Read the model definition and answer for the solid it produces. Units are mm, in the model's axes. A direction names the side the tool comes from. Coordinates: 2 decimals unless noted, no trailing zeros. Use a Markdown table: item, result.
from build123d import *

# Parameters (mm, degrees)
BOSS_EXTRUDE1_DEPTH = 11.1125
SKETCH2_R           = 12
CUT_EXTRUDE1_DEPTH  = 6
SKETCH3_R           = 10
CUT_EXTRUDE2_DEPTH  = 136.768702671
SKETCH4_R           = 3.2639
CUT_EXTRUDE3_DEPTH  = 137.09051503
SKETCH5_R           = 9.525
CUT_EXTRUDE4_DEPTH  = 4.7625
SKETCH6_R           = 2.778125
CUT_EXTRUDE5_DEPTH  = 38.1


with BuildPart() as part:
    # Sketch1 → Boss-Extrude1 (new body)
    with BuildSketch(Plane(origin=(-18.0375, 0, 0), x_dir=(0, 0, -1), z_dir=(1, 0, 0))):
        Polygon((-47.625, -127), (-47.625, 19.726920908), (-19.726920908, 47.625), (19.726920908, 47.625), (47.625, 19.726920908), (47.625, -127), align=None)
    extrude(amount=-BOSS_EXTRUDE1_DEPTH)

    # Sketch2 → Cut-Extrude1 (cut)
    with BuildSketch(Plane(origin=(-18.0375, 0, 0), x_dir=(0, 0, -1), z_dir=(1, 0, 0))):
        with Locations(Location((0, 0, 0), (0, 0, 90))):
            Circle(SKETCH2_R)
    extrude(amount=-CUT_EXTRUDE1_DEPTH, mode=Mode.SUBTRACT)

    # Sketch3 → Cut-Extrude2 (cut, through all)
    with BuildSketch(Plane(origin=(-24.0375, 0, 0), x_dir=(0, 0, -1), z_dir=(1, 0, 0))):
        with Locations(Location((0, 0, 0), (0, 0, 90))):
            Circle(SKETCH3_R)
    extrude(amount=-CUT_EXTRUDE2_DEPTH, mode=Mode.SUBTRACT)

    # Sketch4 → Cut-Extrude3 (cut, through all)
    with BuildSketch(Plane.ZY.offset(29.15)):
        with Locations((0, -31.75)):
            Circle(SKETCH4_R)
        with Locations((31.75, 0)):
            Circle(SKETCH4_R)
        with Locations((-31.75, 0)):
            Circle(SKETCH4_R)
        with Locations((0, 31.75)):
            Circle(SKETCH4_R)
    extrude(amount=-CUT_EXTRUDE3_DEPTH, mode=Mode.SUBTRACT)

    # Sketch5 → Cut-Extrude4 (cut)
    with BuildSketch(Plane(origin=(-18.0375, 0, 0), x_dir=(0, 0, -1), z_dir=(1, 0, 0))):
        with Locations(Location((-31.75, 0, 0), (0, 0, 90))):
            Circle(SKETCH5_R)
        with Locations(Location((0, 31.75, 0), (0, 0, 90))):
            Circle(SKETCH5_R)
        with Locations(Location((31.75, 0, 0), (0, 0, 90))):
            Circle(SKETCH5_R)
        with Locations(Location((0, -31.75, 0), (0, 0, 90))):
            Circle(SKETCH5_R)
    extrude(amount=-CUT_EXTRUDE4_DEPTH, mode=Mode.SUBTRACT)

    # Sketch6 → Cut-Extrude5 (cut)
    with BuildSketch(Plane.XZ.offset(127)):
        with Locations((-23.59375, 0)):
            Circle(SKETCH6_R)
        with Locations((-23.59375, 38.1)):
            Circle(SKETCH6_R)
        with Locations((-23.59375, -38.1)):
            Circle(SKETCH6_R)
    extrude(amount=-CUT_EXTRUDE5_DEPTH, mode=Mode.SUBTRACT)


solid = part.part
(1) Straight lines are drawn through the part: L1, parallel to Z at x = -21.4, y = 0 (3 decimals); L2, parallel to Z at x = -23, y = 0.5 (3 decimals); L3, parallel to X at y = 28, z = 6. For each, find the intervals that lie inside material, in ascending order.
Report:
| item | result |
|---|---|
| L1 | z = -47.625 to -41.275, -22.225 to -12, 12 to 22.225, 41.275 to 47.625 |
| L2 | z = -47.625 to -34.975, -28.525 to -11.99, 11.99 to 28.525, 34.975 to 47.625 |
| L3 | x = -29.15 to -22.8 |
(2) A cutting plane is placed at A-A, the plane z = 0. Count the separate pieces of the cut face and the enclosed holes in it, and give its area (3 significant figures).
Report:
| item | result |
|---|---|
| separate pieces | 4 |
| enclosed holes | 0 |
| area | 1,220 mm² |
(3) Each of these flat-tipped pins is pushed along its axis until it touches: P1, Ø22, axis at y = 0, z = -31.75, coming from the -X side; P2, Ø3.5, axis at x = -23.59, z = 38.1, coming from the +Y side; P3, Ø5.5, axis at y = 4, z = 34, coming from the +X side; P4, Ø6, axis at x = -20, z = -33, coming from the +Y side. Where does it stop, or does it pass through?
Report:
| item | result |
|---|---|
| P1 | stops at x = -29.15 |
| P2 | stops at y = 31 |
| P3 | stops at x = -22.8 |
| P4 | stops at y = 37.35 |
(4) The mould has two halves that part along X. Classify faces 1 (the flat face through (-18.038, -58, -1)), 2 (the cylindrical face through (-26.019, 28.564, -0.708)), 3 (the flat face through (-29.15, -38, -1)), 4 (the cylindrical face through (-23.955, -108.217, -35.346)): pulls with the +X half, pulls with the -X half, needs draft (parallel to the pull), parting line crosses it, or undercut.
Report:
| item | result |
|---|---|
| face 1 | pulls with the +X half |
| face 2 | needs draft |
| face 3 | pulls with the -X half |
| face 4 | undercut |
(5) For faces 5 (the flat face through (-24, -55, 47.625)), 6 (the flat face through (-24, -88.9, 0)), 7 (the cylindrical face through (-20.385, 24.191, -5.796)), determine the directions among +Z, -Z, +X, -X, +Y, -Y from which every point of the face is accessible in a straight line to the end or side of a thin tool.
Report:
| item | result |
|---|---|
| face 5 | +Z, +X, -X, +Y, -Y |
| face 6 | -Y |
| face 7 | +X |
